Input: part model. Units: mm. Frame: model coordinates. Give positions to 0.01 mm unless a question says otherwise; leave off trailing zeros. Loops run counter-clockwise (first coordinate to the right, second up) from the corner with the lowest first, then second, coordinate; pieces in that order, holes last.
from build123d import *

# Parameters (mm, degrees)
SKETCH_1_R      = 6
EXTRUDE_1_DEPTH = 11


with BuildPart() as part:
    # 草图1 → 凸台-拉伸1 (new body)
    with BuildSketch(Plane(origin=(0, 0, 0), x_dir=(1, 0, 0), z_dir=(0, 1, 0))):
        Polygon((12.586235868, 0), (6.293117934, 10.9), (-6.293117934, 10.9), (-12.586235868, 0), (-6.293117934, -10.9), (6.293117934, -10.9), align=None)
        with Locations(Location((0, 0, 0), (0, 0, 270))):
            Circle(SKETCH_1_R, mode=Mode.SUBTRACT)
    extrude(amount=EXTRUDE_1_DEPTH)

    # 草图2 → 切除-旋转3 (revolve, cut)
    with BuildSketch(Plane.XY):
        Polygon((12.586235868, 10), (9.586235868, 11), (12.586235868, 11), align=None)
        Polygon((12.586235868, 1), (9.586235868, 0), (12.586235868, 0), align=None)
    revolve(axis=Axis((0, 0, 0), (0, 1, 0)), mode=Mode.SUBTRACT)


solid = part.part
(1) Pin query (flat end, axial travel): pin 1 Ø1.5 at (y, z) = (6, 3.5) entering from +X; pin 2 Ø4 at (y, z) = (4, -4) entering from +X; pin 3 Ø1 at (y, z) = (4.5, 2) entering from -X; pin 4 Ø7 at (x, z) = (0, 0) entering from -Y. Return the tip coordinate at first contact, or that it passes through.
Values follow:
pin 1: stops at x = 11
pin 2: stops at x = 11.43
pin 3: stops at x = -11.72
pin 4: passes through
(2) Cut plane A-A (x = 0). Return the cut outline in (y, z).
Values follow:
outline: (0, -9.59) - (0.44, -10.9) - (10.56, -10.9) - (11, -9.59) - (11, -6) - (0, -6) - close; (0, 6) - (11, 6) - (11, 9.59) - (10.56, 10.9) - (0.44, 10.9) - (0, 9.59) - close
(3) Mould query, pull axis Z, two halves, no side actions, for faces 1 (the flat face through (-9.484, 5.429, 5.374)), 2 (the conical face through (-9.722, 0.049, -0.428)), 3 (the cylindrical face through (1.802, 5.423, 5.723)). Classes: +Z half, -Z half, draft (parallel to the pull), parting line (faces both ways), or undercut.
Values follow:
face 1: +Z half
face 2: parting line
face 3: undercut
(4) Cut plane B-B (y = 6). Return the cut outline in (x, z).
Values follow:
outline: (-12.59, 0) - (-6.29, -10.9) - (6.29, -10.9) - (12.59, 0) - (6.29, 10.9) - (-6.29, 10.9) - close; hole circle Ø12 at (0, 0)
(5) Ray query, probe 1 along X at (y, z) = (6, -5); probe 2 along Z at (x, y) = (2.5, 4); probe 3 along Z at (x, y) = (1.75, 2.25). Return the intervals inside material, ascending.
Values follow:
probe 1: x = -9.7 to -3.32, 3.32 to 9.7
probe 2: z = -10.9 to -5.45, 5.45 to 10.9
probe 3: z = -10.9 to -5.74, 5.74 to 10.9
